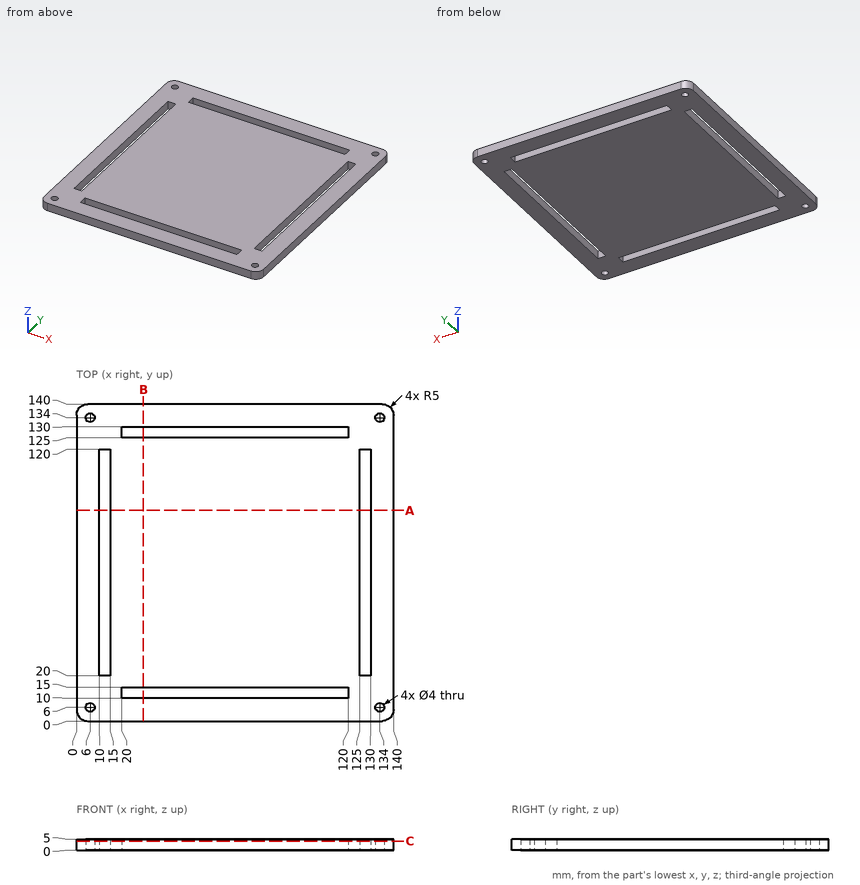
Check sheet for the drawn part. Datum: minimum x, y, z corner. Units: mm. Round coordinates to 2 decimals unless told otherwise and drop trailing zeros. Order: outer loops, then holes, each group sorted by start corner. A loop starts at its lowest first (then second) coordinate and runs counter-clockwise, first axis right, second up.
(1) Cross-section at A-A, the plane y = 93. Enter the section's corners in (x, z).
(2) Cross-section at C-C, the plane z = 4.05. State how many separate pieces and enclosed holes the cut face has, and give its area (3 significant figures).
(3) Scan lines: probe 1 along X at (y, z) = (6, 2.75); probe 2 along X at (y, z) = (93.5, 4.55). Record each from-to range of solid material in increasing order.
(4) Go/stop test with a flat-tipped pin: P1, Ø3.5, axis at x = 134, y = 6, coming from the -Z side. Record where the tip stops, or that it passes through.
Check sheet entries:
1. outline: (0, 0) - (10, 0) - (10, 5) - (0, 5) - close; (15, 0) - (125, 0) - (125, 5) - (15, 5) - close; (130, 0) - (140, 0) - (140, 5) - (130, 5) - close
2. separate pieces: 1
2. enclosed holes: 8
2. area: 17,500 mm2
3. probe 1: x = 0 to 4, 8 to 132, 136 to 140
3. probe 2: x = 0 to 10, 15 to 125, 130 to 140
4. P1: passes through
